Autodesk Inventor part; units mm, degrees
ref_plane "YZ Plane" through (0, 0, 0) normal (1, 0, 0) x (0, 1, 0)
ref_plane "XZ Plane" through (0, 0, 0) normal (0, 1, 0) x (-1, 0, 0)
ref_plane "XY Plane" through (0, 0, 0) normal (0, 0, 1) x (1, 0, 0)
sketch "T-Slot 4040 Base" plane through (0, 0, 0) normal (0, 0, 1) x (1, 0, 0)
  line L0 (-28, 0) -> (28, 0) construction
  line L1 (0, -28) -> (0, 28) construction
  circle A0 centre (0, 0) radius 5.1
  line L2 (-7.5, -7.5) -> (7.5, -7.5)
  line L3 (7.5, -7.5) -> (7.5, 7.5)
  line L4 (7.5, 7.5) -> (-7.5, 7.5)
  line L5 (-7.5, 7.5) -> (-7.5, -7.5)
  line L6 (-7.5, -7.5) -> (7.5, 7.5) construction
  line L7 (7.5, -7.5) -> (-7.5, 7.5) construction
  line L8 (-20, 20) -> (20, 20)
  line L9 (20, 20) -> (20, -20)
  line L10 (20, -20) -> (-20, -20)
  line L11 (-20, -20) -> (-20, 20)
  line L12 (-20, 20) -> (20, -20) construction
  line L13 (20, 20) -> (-20, -20) construction
  line L14 (20, 5) -> (14.5, 5)
  line L15 (14.5, 5) -> (14.5, 10)
  line L16 (14.5, 10) -> (12.4749, 10)
  line L17 (12.4749, 10) -> (7.5, 5.0251)
  line L18 (5, 20) -> (5, 14.5)
  line L19 (5, 14.5) -> (10, 14.5)
  line L20 (10, 14.5) -> (10, 12.4749)
  line L21 (10, 12.4749) -> (5.0251, 7.5)
  line L22 (18.5, 18.5) -> (11.5, 18.5)
  line L23 (11.5, 18.5) -> (11.5, 11.5)
  line L24 (11.5, 11.5) -> (18.5, 11.5)
  line L25 (18.5, 11.5) -> (18.5, 18.5)
  line L26 (18.5, 18.5) -> (11.5, 11.5) construction
  line L27 (11.5, 18.5) -> (18.5, 11.5) construction
  line L28 (3.0732, 1.3088) -> (4.38, 2.6125) construction
  line L29 (5.905, 4.1338) -> (4.1393, 5.9037)
  line L30 (4.1393, 5.9037) -> (2.6122, 4.3802)
  line L31 (1.3075, 3.0787) -> (3.0732, 1.3088) construction
  line L32 (3.0732, 1.3088) -> (4.1393, 5.9037) construction
  line L33 (5.905, 4.1338) -> (1.3075, 3.0787) construction
  line L34 (4.38, 2.6125) -> (5.905, 4.1338)
  line L35 (2.6122, 4.3802) -> (1.3075, 3.0787) construction
  line L36 (-20, 5) -> (-14.5, 5)
  line L37 (-14.5, 5) -> (-14.5, 10)
  line L38 (-14.5, 10) -> (-12.4749, 10)
  line L39 (-12.4749, 10) -> (-7.5, 5.0251)
  line L40 (-5, 20) -> (-5, 14.5)
  line L41 (-5, 14.5) -> (-10, 14.5)
  line L42 (-10, 14.5) -> (-10, 12.4749)
  line L43 (-10, 12.4749) -> (-5.0251, 7.5)
  line L44 (-18.5, 18.5) -> (-11.5, 18.5)
  line L45 (-11.5, 18.5) -> (-11.5, 11.5)
  line L46 (-11.5, 11.5) -> (-18.5, 11.5)
  line L47 (-18.5, 11.5) -> (-18.5, 18.5)
  line L48 (-5.905, 4.1338) -> (-4.1393, 5.9037)
  line L49 (-4.1393, 5.9037) -> (-2.6122, 4.3802)
  line L50 (-4.38, 2.6125) -> (-5.905, 4.1338)
  line L51 (7.5, -7.5) -> (-7.5, -7.5)
  line L52 (20, -5) -> (14.5, -5)
  line L53 (14.5, -5) -> (14.5, -10)
  line L54 (14.5, -10) -> (12.4749, -10)
  line L55 (12.4749, -10) -> (7.5, -5.0251)
  line L56 (5, -20) -> (5, -14.5)
  line L57 (5, -14.5) -> (10, -14.5)
  line L58 (10, -14.5) -> (10, -12.4749)
  line L59 (10, -12.4749) -> (5.0251, -7.5)
  line L60 (18.5, -18.5) -> (11.5, -18.5)
  line L61 (11.5, -18.5) -> (11.5, -11.5)
  line L62 (11.5, -11.5) -> (18.5, -11.5)
  line L63 (18.5, -11.5) -> (18.5, -18.5)
  line L64 (18.5, -18.5) -> (11.5, -11.5) construction
  line L65 (11.5, -18.5) -> (18.5, -11.5) construction
  line L66 (3.0732, -1.3088) -> (4.38, -2.6125) construction
  line L67 (5.905, -4.1338) -> (4.1393, -5.9037)
  line L68 (4.1393, -5.9037) -> (2.6122, -4.3802)
  line L69 (1.3075, -3.0787) -> (3.0732, -1.3088) construction
  line L70 (3.0732, -1.3088) -> (4.1393, -5.9037) construction
  line L71 (5.905, -4.1338) -> (1.3075, -3.0787) construction
  line L72 (4.38, -2.6125) -> (5.905, -4.1338)
  line L73 (2.6122, -4.3802) -> (1.3075, -3.0787) construction
  line L74 (-4.38, -2.6125) -> (-5.905, -4.1338)
  line L75 (-4.1393, -5.9037) -> (-2.6122, -4.3802)
  line L76 (-5.905, -4.1338) -> (-4.1393, -5.9037)
  line L77 (-12.4749, -10) -> (-7.5, -5.0251)
  line L78 (-10, -12.4749) -> (-5.0251, -7.5)
  line L79 (-10, -14.5) -> (-10, -12.4749)
  line L80 (-5, -14.5) -> (-10, -14.5)
  line L81 (-5, -20) -> (-5, -14.5)
  line L82 (-18.5, -18.5) -> (-11.5, -18.5)
  line L83 (-11.5, -18.5) -> (-11.5, -11.5)
  line L84 (-11.5, -11.5) -> (-18.5, -11.5)
  line L85 (-18.5, -11.5) -> (-18.5, -18.5)
  line L86 (-14.5, -10) -> (-12.4749, -10)
  line L87 (-14.5, -5) -> (-14.5, -10)
  line L88 (-20, -5) -> (-14.5, -5)
  point P0 (15, 15)
  point P1 (3.6062, 3.6062)
  point P2 (3.6062, 3.6062)
  point P3 (15, -15)
  point P4 (3.6062, -3.6062)
  point P5 (3.6062, -3.6062)
  dimension "d9" = 10.2
  dimension "d12" = 40
  dimension "d13" = 40
  dimension "d14" = 5.5
  dimension "d15" = 15
  dimension "d16" = 7
  dimension "d17" = 10
  dimension "d20" = 1.75
  dimension "d21" = 7
  dimension "d22" = 2
  dimension "d29" = 1.5
  dimension "d30" = 2.5
extrude "Extrusion1" add sketch "T-Slot 4040 Base" along normal blind 1207 contours L5 L4 L3 L2 | L2 L78 L79 L80 L81 L10 L11 L88 L87 L86 L77 L5 | L2 L3 L55 L54 L53 L52 L9 L10 L56 L57 L58 L59 | L39 L38 L37 L36 L11 L8 L40 L41 L42 L43 L4 L5 | L3 L4 L21 L20 L19 L18 L8 L9 L14 L15 L16 L17
fillet "Rundung1" radius 1 16 edges at (11.5, 18.5, 603.5) (18.5, 18.5, 603.5) (18.5, 11.5, 603.5) (11.5, 11.5, 603.5) (-11.5, 18.5, 603.5) (-18.5, 18.5, 603.5) (-18.5, 11.5, 603.5) (-11.5, 11.5, 603.5) (-18.5, -11.5, 603.5) (-11.5, -11.5, 603.5) (-11.5, -18.5, 603.5) (-18.5, -18.5, 603.5) (11.5, -18.5, 603.5) (11.5, -11.5, 603.5) (18.5, -11.5, 603.5) (18.5, -18.5, 603.5)
fillet "Rundung2" radius 3 4 edges at (20, 20, 603.5) (20, -20, 603.5) (-20, -20, 603.5) (-20, 20, 603.5)
properties part number "T-SLOT 4040 B-Type 1207mm"
Input: part model. Units: mm. Frame: model coordinates. Coordinates: 2 decimals unless noted, no trailing zeros. Use a Markdown table: item, result. Add a question column.
1) Pin query (flat end, axial travel): P1, Ø6, axis at x = -4.5, z = 505.5, coming from the +Y side; P2, Ø5, axis at x = -2, z = 1042, coming from the +Y side. Return the tip coordinate at first contact, or that it passes through.
2) Line query: L1, parallel to X at y = -15, z = 336.5; L2, parallel to Y at x = 13.5, z = 75.5. Output: solid intervals per line, ascending. Write a range as from..to.
3) Section A-A, the plane z = 759.5. Give the number of separate pieces and of enclosed holes in the cut face, plus the area to 3 significant figures.
Answer below:
| question | item | result |
|---|---|---|
| 1 | P1 | y = 20 |
| 1 | P2 | y = 7.5 |
| 2 | L1 | -20..-18.5, -11.5..-5, 5..11.5, 18.5..20 |
| 2 | L2 | -20..-18.5, -11.5..-10, 10..11.5, 18.5..20 |
| 3 | separate pieces | 1 |
| 3 | enclosed holes | 5 |
| 3 | area | 616 mm2 |
